Source: CAD feature listing. Evaluate the final solid. Frame: model axes, mm. Give positions to 0.01 mm unless a question says otherwise; leave off trailing zeros. Write each loop counter-clockwise with the first axis right and the second up, starting at its lowest first coordinate (ties: lowest second). Pieces come first, ordered by that corner, then holes. Notation, with made-up numbers: M -25.5,84 L -6.5,84 A15 ccw -6.5,104 Z; hole C 68,85.25 d2. An arc over 180 degrees is marked long. Return JSON: item names as keys, results as strings.
```python
from build123d import *

# Parameters (mm, degrees)
SKETCH_1_R      = 5
EXTRUDE_1_DEPTH = 2


with BuildPart() as part:
    # 草图1 → 凸台-拉伸1 (new, symmetric)
    with BuildSketch(Plane.XY):
        with BuildLine():
            Line((10, 0), (110, 0))
            ThreePointArc((110, 0), (117.071067812, -2.928932188), (120, -10))
            Line((120, -10), (120, -90))
            ThreePointArc((120, -90), (102.426406871, -132.426406871), (60, -150))
            ThreePointArc((60, -150), (17.573593129, -132.426406871), (0, -90))
            Line((0, -90), (0, -10))
            ThreePointArc((0, -10), (2.928932188, -2.928932188), (10, 0))
        make_face()
        with Locations((60, -130)):
            Circle(SKETCH_1_R, mode=Mode.SUBTRACT)
        with Locations((60, -110)):
            Circle(SKETCH_1_R, mode=Mode.SUBTRACT)
        with Locations((60, -90)):
            Circle(SKETCH_1_R, mode=Mode.SUBTRACT)
    extrude(amount=EXTRUDE_1_DEPTH, both=True)


solid = part.part
```
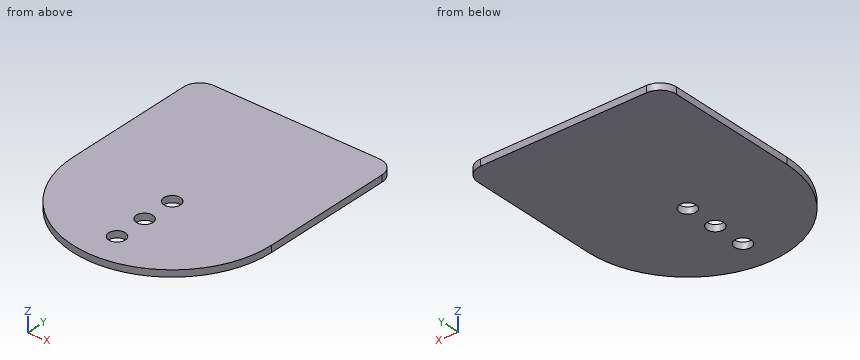
1) Cut plane A-A, the plane x = 60. Return the cut outline in (y, z), then the cut area to 3 significant figures.
Numbers:
{"outline": "M -150,-2 L -135,-2 L -135,2 L -150,2 Z; M -125,-2 L -115,-2 L -115,2 L -125,2 Z; M -105,-2 L -95,-2 L -95,2 L -105,2 Z; M -85,-2 L 0,-2 L 0,2 L -85,2 Z", "area": "480 mm²"}
2) Contact query for a flat-ended pin moving along its axis: pin 1 Ø1 at (y, z) = (-123, 0) entering from +X. Output: stop coordinate, or through.
Numbers:
{"pin 1": "stops at x = 110.44"}
3) Cut plane D-D, the plane y = -110. Return the cut outline in (x, z).
Numbers:
{"outline": "M 3.43,-2 L 55,-2 L 55,2 L 3.43,2 Z; M 65,-2 L 116.57,-2 L 116.57,2 L 65,2 Z"}
4) Cut plane B-B, the plane z = 1.3. Return the cut outline in (x, y), then the cut area to 3 significant figures.
Numbers:
{"outline": "M 0,-90 A60 ccw 120,-90 L 120,-10 A10 ccw 110,0 L 10,0 A10 ccw 0,-10 Z; hole C 60,-130 d10; hole C 60,-110 d10; hole C 60,-90 d10", "area": "16,200 mm²"}
5) Line query: line 1 (Y direction, x = 60, z = 1.25); line 2 (Y direction, x = 64.5, z = -0.55); line 3 (X direction, y = -90.5, z = 0). Output: solid intervals per line, ascending. Write a range as [from, to].
Numbers:
{"line 1": "y = [-150, -135], [-125, -115], [-105, -95], [-85, 0]", "line 2": "y = [-149.83, -132.18], [-127.82, -112.18], [-107.82, -92.18], [-87.82, 0]", "line 3": "x = [0, 55.03], [64.97, 120]"}
6) Cut plane C-C, the plane y = -130. Return the cut outline in (x, z).
Numbers:
{"outline": "M 15.28,-2 L 55,-2 L 55,2 L 15.28,2 Z; M 65,-2 L 104.72,-2 L 104.72,2 L 65,2 Z"}
